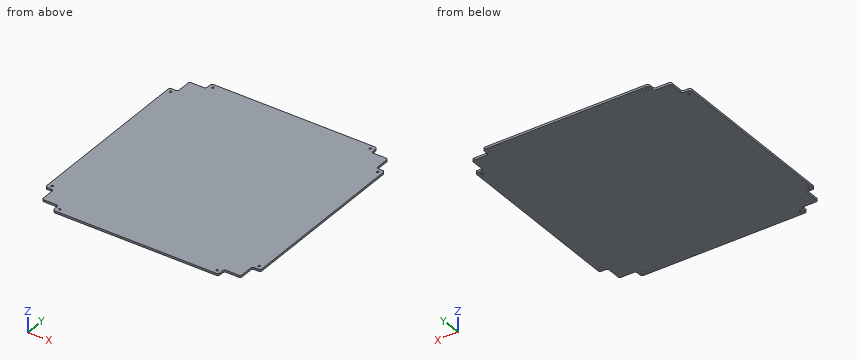
```python
from build123d import *

# Parameters (mm, degrees)
SKETCH_1_W          = 520
SKETCH_1_H          = 550
EXTRUDE_1_DEPTH     = 5
SKETCH_2_R          = 2.5
CUT_EXTRUDE_2_DEPTH = 379.483817356
FILLET_2_R          = 5


with BuildPart() as part:
    # 草图1 → 凸台-拉伸1 (new body)
    with BuildSketch(Plane.XY):
        Rectangle(SKETCH_1_W, SKETCH_1_H)
    extrude(amount=EXTRUDE_1_DEPTH)

    # 草图2 → 切除-拉伸2 (cut, through all)
    with BuildSketch(Plane.XY.offset(5)):
        with Locations((-190, 265)):
            Circle(SKETCH_2_R)
        with Locations((190, 265)):
            Circle(SKETCH_2_R)
        with Locations((250, 205)):
            Circle(SKETCH_2_R)
        with Locations((-250, 205)):
            Circle(SKETCH_2_R)
        with Locations((-250, -205)):
            Circle(SKETCH_2_R)
        with Locations((-190, -265)):
            Circle(SKETCH_2_R)
        with Locations((190, -265)):
            Circle(SKETCH_2_R)
        with Locations((250, -205)):
            Circle(SKETCH_2_R)
        Polygon((240, 255), (200, 255), (200, 275), (260, 275), (260, 215), (240, 215), align=None)
        Polygon((-240, 255), (-240, 215), (-260, 215), (-260, 275), (-200, 275), (-200, 255), align=None)
        Polygon((-240, -255), (-200, -255), (-200, -275), (-260, -275), (-260, -215), (-240, -215), align=None)
        Polygon((240, -255), (240, -215), (260, -215), (260, -275), (200, -275), (200, -255), align=None)
    extrude(amount=-CUT_EXTRUDE_2_DEPTH, mode=Mode.SUBTRACT)

    # 圆角2
    fillet_2_edges = [part.edges().sort_by_distance(p)[0] for p in [
        (260, 215, 2.5),
        (240, 215, 2.5),
        (240, 255, 2.5),
        (200, 255, 2.5),
        (200, 275, 2.5),
        (-200, 275, 2.5),
        (-200, 255, 2.5),
        (-240, 255, 2.5),
        (-240, 215, 2.5),
        (-260, 215, 2.5),
        (-260, -215, 2.5),
        (-240, -215, 2.5),
        (-240, -255, 2.5),
        (-200, -255, 2.5),
        (-200, -275, 2.5),
        (200, -275, 2.5),
        (200, -255, 2.5),
        (240, -255, 2.5),
        (240, -215, 2.5),
        (260, -215, 2.5),
    ]]
    fillet(fillet_2_edges, radius=FILLET_2_R)


solid = part.part
```
Read the model definition and answer for the solid it produces. Units are mm, in the model's axes. Coordinates: 2 decimals unless noted, no trailing zeros. Write each loop counter-clockwise with the first axis right and the second up, starting at its lowest first coordinate (ties: lowest second). Pieces come first, ordered by that corner, then holes. Notation, with made-up numbers: (-39.5, 30.25) - (-13.5, 30.25) arc R20 cw to (-13.5, 35.25) - close; hole circle Ø11 at (15, 77.5). An arc over 180 degrees is marked (long way). Answer as a JSON object with one key per item and string values. Group by question number.
1. A cutting plane is placed at A-A (y = -228). Determine the outline of the cut face in (x, z), plus the area to 3 significant figures.
2. Consider L1, parallel to Y at x = -190, z = 2.6; L2, parallel to X at y = 265, z = 2.3; L3, parallel to X at y = -205, z = 3.2. Determine where each line is inside the solid, lowest interval first. Write a range as [from, to].
3. A cutting plane is placed at B-B (z = 2.8). Give the number of separate pieces and of enclosed holes in the cut face, plus the area to 3 significant figures.
4. Each of these flat-tipped pins is pushed along its axis until it touches: P1, Ø2.5, axis at x = -213, z = 3, coming from the +Y side; P2, Ø4, axis at x = 190, y = 265, coming from the -Z side; P3, Ø2.5, axis at x = -250, z = 3, coming from the +Y side; P4, Ø1.5, axis at x = -251.5, z = 3.5, coming from the -Y side. Where does it stop, or does it pass through?
Worked out:
{
 "1": {"outline": "(-240, 0) - (240, 0) - (240, 5) - (-240, 5) - close", "area": "2,400 mm²"},
 "2": {"L1": "y = [-275, -267.5], [-262.5, 262.5], [267.5, 275]", "L2": "x = [-200, -192.5], [-187.5, 187.5], [192.5, 200]", "L3": "x = [-260, -252.5], [-247.5, 247.5], [252.5, 260]"},
 "3": {"separate pieces": "1", "enclosed holes": "8", "area": "278,000 mm²"},
 "4": {"P1": "stops at y = 255", "P2": "passes through", "P3": "stops at y = 215", "P4": "stops at y = -215"}
}
